from build123d import *

# Parameters (mm, degrees)
SKETCH1_W           = 38.1
SKETCH1_H           = 38.1
SKETCH1_R           = 2.54
SKETCH1_R_2         = 3.81
BOSS_EXTRUDE1_DEPTH = 3.175
FILLET1_R           = 2.54


with BuildPart() as part:
    # Sketch1 → Boss-Extrude1 (new body)
    with BuildSketch(Plane(origin=(0, 0, 0), x_dir=(1, 0, 0), z_dir=(0, 1, 0))):
        Rectangle(SKETCH1_W, SKETCH1_H)
        with Locations((9.525, 9.525)):
            Circle(SKETCH1_R, mode=Mode.SUBTRACT)
        with Locations((-9.525, -9.525)):
            Circle(SKETCH1_R, mode=Mode.SUBTRACT)
        Circle(SKETCH1_R_2, mode=Mode.SUBTRACT)
    extrude(amount=BOSS_EXTRUDE1_DEPTH)

    # Fillet1
    fillet1_edges = [part.edges().sort_by_distance(p)[0] for p in [
        (-19.05, 1.5875, -19.05),
        (19.05, 1.5875, -19.05),
        (19.05, 1.5875, 19.05),
        (-19.05, 1.5875, 19.05),
    ]]
    fillet(fillet1_edges, radius=FILLET1_R)


solid = part.part
The model under review builds one solid part; all positions refer to its coordinate system, in mm. Give positions to 0.01 mm unless a question says otherwise; leave off trailing zeros. Order: outer loops, then holes, each group sorted by start corner. A loop starts at its lowest first (then second) coordinate and runs counter-clockwise, first axis right, second up. Notation, with made-up numbers: M 83,35.5 L 103,35.5 A11 ccw 103,42.5 Z; hole C -12.5,-5 d10. An arc over 180 degrees is marked long. Answer in a Markdown table with one row per item. Add a question column.
1. To check wall thickness, follow line 1 along X through (y, z) = (2.2, -0.5); line 2 along X through (y, z) = (2.05, 11); line 3 along Z through (x, y) = (11.5, 0.1). State the ranges of each line that lie inside material, in increasing order.
2. For pin 1 Ø4 at (x, z) = (-9.525, 9.525) entering from +Y, flat-tipped, find the tip position at first contact; note if it passes through.
3. Add section A-A on z = 0. State the section outline as (x, y) points (3 decimals).
4. Add section C-C on y = 1.9. State the section outline as (x, z) points (3 decimals).
5. Mouldability with a two-part tool opening along X and no side actions: class faces 1 (the cylindrical face through (-0.83, 1.57, 3.72)), 2 (the cylindrical face through (7.51, 1.57, -7.98)), 3 (the cylindrical face through (18.286, 1.61, 18.326)), 4 (the flat face through (0, 2, 19.05)) as released by +X, released by -X, zero draft, split by the parting line, or undercut.
6. Add section B-B on x = 0. State the section outline as (y, z) points (3 decimals), plus the area to 3 significant figures.
The answers:
| question | item | result |
|---|---|---|
| 1 | line 1 | -19.05 to -3.78, 3.78 to 19.05 |
| 1 | line 2 | -19.05 to -11.59, -7.46 to 19.05 |
| 1 | line 3 | -19.05 to -11.12, -7.93 to 19.05 |
| 2 | pin 1 | through |
| 3 | outline | M -19.05,0 L -3.81,0 L -3.81,3.175 L -19.05,3.175 Z; M 3.81,0 L 19.05,0 L 19.05,3.175 L 3.81,3.175 Z |
| 4 | outline | M -19.05,-16.51 A2.54 ccw -16.51,-19.05 L 16.51,-19.05 A2.54 ccw 19.05,-16.51 L 19.05,16.51 A2.54 ccw 16.51,19.05 L -16.51,19.05 A2.54 ccw -19.05,16.51 Z; hole C -9.525,9.525 d5.08; hole C 0,0 d7.62; hole C 9.525,-9.525 d5.08 |
| 5 | face 1 | undercut |
| 5 | face 2 | undercut |
| 5 | face 3 | released by +X |
| 5 | face 4 | zero draft |
| 6 | outline | M 0,-19.05 L 3.175,-19.05 L 3.175,-3.81 L 0,-3.81 Z; M 0,3.81 L 3.175,3.81 L 3.175,19.05 L 0,19.05 Z |
| 6 | area | 96.8 mm2 |
